from build123d import *

# Parameters (mm, degrees)
SKETCH001_W     = 3.4
SKETCH001_H     = 4.2
POCKET_DEPTH    = 5
POCKET001_DEPTH = 1.3


with BuildPart() as part:
    # Sketch → Revolution (revolve)
    with BuildSketch(Plane.XZ):
        with BuildLine():
            Line((0, 1.9), (-2.1, 1.9))
            ThreePointArc((-2.1, 1.9), (-2.382843, 1.782843), (-2.5, 1.5))
            Line((-2.5, 1.5), (-2.5, 0))
            Line((-2.5, 0), (-4, 0))
            Line((-4, 0), (-4, -1.2))
            ThreePointArc((-4, -1.4), (-3.9, -1.3), (-4, -1.2))
            Line((-4, -1.4), (-4, -2.3))
            Line((-4, -2.3), (-5.555606, -4.521636))
            ThreePointArc((-5.555606, -4.521636), (-5.59702, -4.708442), (-5.494212, -4.869818))
            Line((-5.494212, -4.869818), (-5.084636, -5.156606))
            ThreePointArc((-5.084636, -5.156606), (-4.89783, -5.19802), (-4.736454, -5.095212))
            Line((-4.736454, -5.095212), (-2.919267, -2.5))
            Line((-2.919267, -2.5), (0, -2.5))
            Line((0, -2.5), (0, 1.9))
        make_face()
    revolve(axis=Axis((0, 0, 0), (0, 0, 1)))

    # Sketch001 → Pocket (cut)
    with BuildSketch(Plane.XY.offset(-1.5)):
        Rectangle(SKETCH001_W, SKETCH001_H)
    extrude(amount=-POCKET_DEPTH, mode=Mode.SUBTRACT)

    # Sketch002 → Pocket001 (cut)
    with BuildSketch(Plane.XY.offset(-0.4)):
        Polygon((-4.3, 1.6), (-4.3, -1.6), (0.7, -1.6), (0.7, -1.1), (1.2, -1.1), (1.2, 1.1), (0.7, 1.1), (0.7, 1.6), align=None)
    extrude(amount=-POCKET001_DEPTH, mode=Mode.SUBTRACT)


solid = part.part
Source: CAD feature listing. Evaluate the final solid. Frame: model axes, mm. A direction names the side the tool comes from. Round coordinates to 2 decimals unless told otherwise and drop trailing zeros. Loops run counter-clockwise (first coordinate to the right, second up) from the corner with the lowest first, then second, coordinate; pieces in that order, holes last.
Q1. Access query for faces 1 (the face through (-1, 1.6, -1)), 2 (the face through (0.54, 2.44, 0.74)), 3 (the face through (1.2, 0, -1)). Directions: +Z, -Z, +X, -X, +Y, -Y. A direction counts if a zero-diameter tool reaches every point of the face in a straight line with its end or side. Return the directions, or none.
Q2. First-contact query: P1, Ø2.5, axis at x = 0.5, y = 1, coming from the -Z side; P2, Ø6.5, axis at x = 0, y = 1, coming from the -Z side; P3, Ø0.6, axis at x = 1, z = -1, coming from the +Y side. Flat tips, straight axial feed; report the tip coordinate or a pass-through.
Q3. Section C-C, the plane z = 1.25. Return loops of the section in (x, y).
Q4. Ray query, line 1 (Z direction, x = -2, y = 0); line 2 (X direction, y = 2.5, z = -3.75); line 3 (X direction, y = 2, z = -3.25). Return the intervals inside material, ascending.
Q5. Mould query, pull axis Y, two halves, no side actions, for faces 4 (the face through (-1.7, 0, -2)), 5 (the face through (2, -2, 0)), 6 (the face through (4, 0, -2)). Classes: pulls with the +Y half, pulls with the -Y half, needs draft (parallel to the pull), parting line crosses it, or undercut.
Q6. Section D-D, the plane z = -4.25. Return loops of the section in (x, y).
Solutions:
1. face 1: -X
1. face 2: +Z
1. face 3: -Z, -X
2. P1: stops at z = -2.5
2. P2: stops at z = -4.4
2. P3: stops at y = 3.94
3. outline: circle Ø5 at (0, 0)
4. line 1: z = -2.5 to -1.7, -0.4 to 1.9
4. line 2: x = -4.35 to -2.85, 2.85 to 4.35
4. line 3: x = -4.21 to -2.8, 2.8 to 4.21
5. face 4: undercut
5. face 5: needs draft
5. face 6: parting line crosses it
6. outline: circle Ø10.73 at (0, 0); hole circle Ø8.29 at (0, 0)
